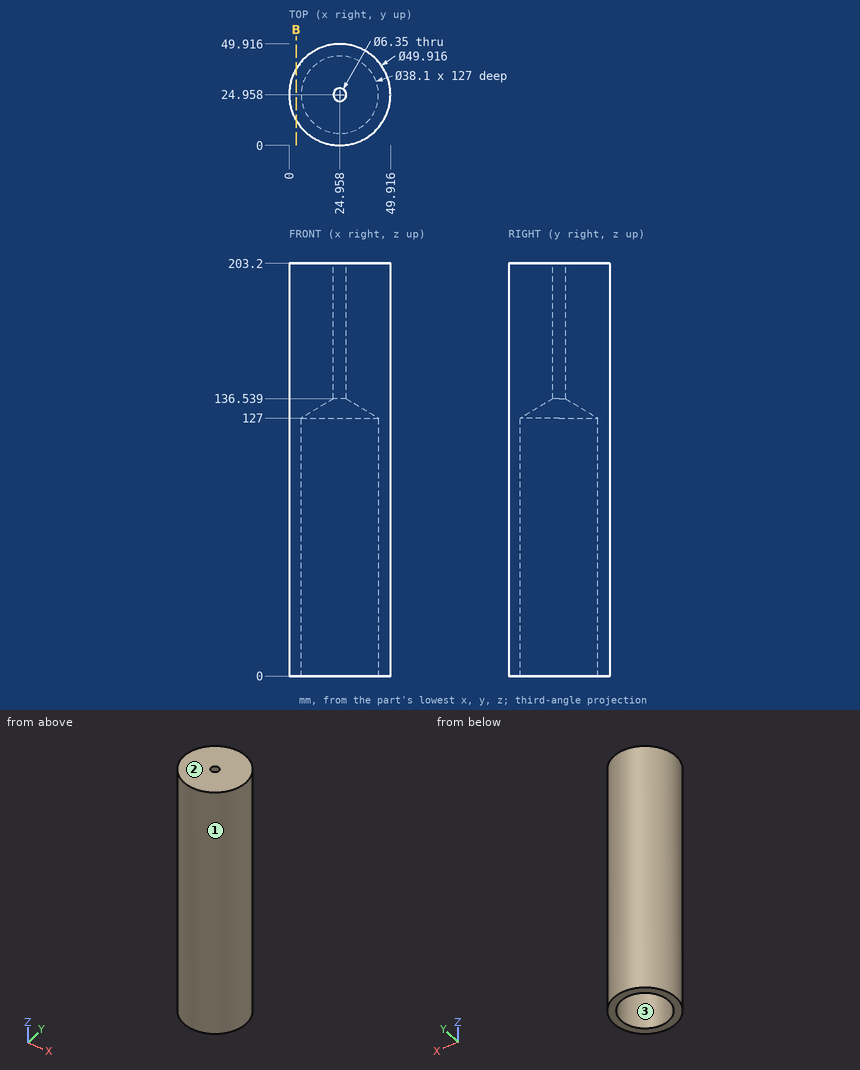
Design review of the part shown in the three views and the two pictorial views. Dimensions are in mm from the part's minimum x, y and z. Give positions to 0.01 mm unless a question says otherwise; leave off trailing zeros. Loops run counter-clockwise (first coordinate to the right, second up) from the corner with the lowest first, then second, coordinate; pieces in that order, holes last. Notation, with made-up numbers: (42.25, 60.25) -> (72.25, 60.25) arc R30 ccw to (72.25, 85.25) -> close; hole circle Ø1 at (14, -5). An arc over 180 degrees is marked (long way). Put each result on its own line as item: value. Start each with the question number.
1. We need section B-B on x = 3.5. State the section outline as (y, z) points.
2. Wall thickness on probe 1 along X at (y, z) = (26, 71.5); probe 2 along Y at (x, z) = (16, 17) (1 decimal); probe 3 along X at (y, z) = (20.5, 35.5) (1 decimal): over which ranges is each line inside the solid? List them lowest first.
3. Clearance check with flat-ended pins moving along their axes: P1, Ø8, axis at x = 28.5, y = 15, coming from the -Z side; P2, Ø5, axis at y = 12.5, z = 171.5, coming from the +X side; P3, Ø5, axis at x = 5, z = 167.5, coming from the +Y side (1 decimal); P4, Ø6, axis at y = 26.5, z = 134.5, coming from the +X side. State where each tip first meets the part, or that it passes through.
4. Mouldability with a two-part tool opening along X and no side actions: class the marked faces 1, 2 and 3 as released by +X, released by -X, zero draft, split by the parting line, or undercut.
Determined:
1. outline: (12.21, 0) -> (37.7, 0) -> (37.7, 203.2) -> (12.21, 203.2) -> close
2. probe 1: 0.02 to 5.94, 43.98 to 49.89
2. probe 2: 1.7 to 8.1, 41.8 to 48.3
2. probe 3: 0.4 to 6.4, 43.5 to 49.5
3. P1: z = 129.69
3. P2: x = 47.84
3. P3: y = 42.8
3. P4: x = 49.92
4. face 1: split by the parting line
4. face 2: zero draft
4. face 3: undercut
